Model file for the job. Use its own axes, mm. A direction names the side the tool comes from. Round coordinates to 2 decimals unless told otherwise and drop trailing zeros. Loops run counter-clockwise (first coordinate to the right, second up) from the corner with the lowest first, then second, coordinate; pieces in that order, holes last.
from build123d import *

# Parameters (mm, degrees)
F1_DEPTH = 70
F2_W     = 20
F2_H     = 15
F3_DEPTH = 25
F4_R     = 5
F5_DEPTH = 70.001


with BuildPart() as f1:
    # F0 (on Front) → F1 (new body)
    with BuildSketch(Plane.XZ):
        Polygon((0, 50), (0, 0), (50, 0), (50, 10), (15, 10), (15, 30), (30, 30), (30, 50), align=None)
    extrude(amount=F1_DEPTH)

    # F2 (on face) → F3 (cut)
    with BuildSketch(Plane.XY.offset(10)):
        with Locations((40, -47.5)):
            Rectangle(F2_W, F2_H)
    extrude(amount=-F3_DEPTH, mode=Mode.SUBTRACT)

    # F4 (on face) → F5 (cut, through all)
    with BuildSketch(Plane.XZ.offset(70)):
        with Locations((10, 40)):
            Circle(F4_R)
    extrude(amount=-F5_DEPTH, mode=Mode.SUBTRACT)


solid = f1.part
Q1. Slice it at A-A on x = 33. Give the cut face in (y, z), plus the area to 3 significant figures.
Q2. Probe line 1 (Y direction, x = 44, z = 7.5); line 2 (Z direction, x = 10, y = -33); line 3 (X direction, y = -43.5, z = 31). List the from-to ranges inside material, lowest first.
Q3. Slice it at B-B on z = 40. Give the cut face in (x, y), plus the area to 3 significant figures.
Q4. Flat gauge pins, fed straight in: P1, Ø10, axis at x = 8.5, z = 44, coming from the +Y side; P2, Ø6, axis at y = -46.5, z = 18, coming from the +X side; P3, Ø4, axis at x = 34.5, y = -19.5, coming from the +Z side; P4, Ø5, axis at y = -46.5, z = 6.5, coming from the +X side. Where does each tip first touch, or does it go through?
Q5. Slice it at D-D on z = 26. Give the cut face in (x, y), plus the area to 3 significant figures.
Q6. Pull direction Y, two halves, no side cores. Call faces 1 (the face through (13, -35, 44)), 2 (the face through (30, -48, 5)), 3 (the face through (14, -70, 20)), 4 (the face through (40, -40, 5)): pulls with the +Y half, pulls with the -Y half, needs draft (parallel to the pull), parting line crosses it, or undercut.
Q7. Slice it at C-C on y = -45.5. Give the cut face in (x, z).
Q8. Tool access for faces 5 (the face through (25, -35, 0)), 6 (the face through (40, -55, 5)), 7 (the face through (14, 0, 20)), 8 (the face through (30, -35, 40)), 9 (the face through (33, -35, 10)): list every direction of +Z, -Z, +X, -X, +Y, -Y with a clear straight run to the whole face (end or side of a thin tool).
Reply:
1. outline: (-70, 0) - (-55, 0) - (-55, 10) - (-70, 10) - close; (-40, 0) - (0, 0) - (0, 10) - (-40, 10) - close
1. area: 550 mm2
2. line 1: y = -70 to -55, -40 to 0
2. line 2: z = 0 to 35, 45 to 50
2. line 3: x = 0 to 30
3. outline: (0, -70) - (5, -70) - (5, 0) - (0, 0) - close; (15, -70) - (30, -70) - (30, 0) - (15, 0) - close
3. area: 1,400 mm2
4. P1: stops at y = 0
4. P2: stops at x = 15
4. P3: stops at z = 10
4. P4: stops at x = 30
5. outline: (0, -70) - (15, -70) - (15, 0) - (0, 0) - close
5. area: 1,050 mm2
6. face 1: needs draft
6. face 2: undercut
6. face 3: pulls with the -Y half
6. face 4: undercut
7. outline: (0, 0) - (30, 0) - (30, 10) - (15, 10) - (15, 30) - (30, 30) - (30, 50) - (0, 50) - close; hole circle Ø10 at (10, 40)
8. face 5: -Z, +X, -X, +Y, -Y
8. face 6: +Z, -Z, +X
8. face 7: +Z, -Z, +X, -X, +Y
8. face 8: +Z, +X, +Y, -Y
8. face 9: +X, +Y, -Y
